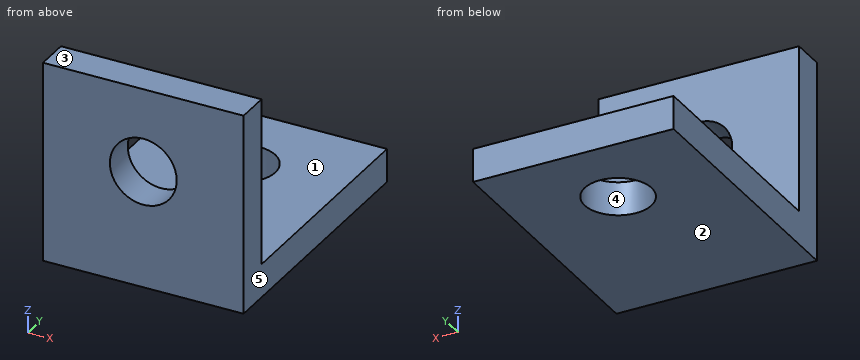
from build123d import *

# Parameters (mm, degrees)
SKETCH1_W           = 19.05
SKETCH1_H           = 19.05
BOSS_EXTRUDE1_DEPTH = 3.175
SKETCH2_W           = 19.05
SKETCH2_H           = 3.175
BOSS_EXTRUDE2_DEPTH = 22.225
CUT_EXTRUDE1_REACH  = 36.925
SKETCH3_R           = 3.175
CUT_EXTRUDE2_REACH  = 37.498
SKETCH4_R           = 3.175


with BuildPart() as part:
    # Sketch1 → Boss-Extrude1 (new body)
    with BuildSketch(Plane(origin=(0, 0, 0), x_dir=(1, 0, 0), z_dir=(0, 1, 0))):
        with Locations((9.525, -9.525)):
            Rectangle(SKETCH1_W, SKETCH1_H)
    extrude(amount=BOSS_EXTRUDE1_DEPTH)

    # Sketch2 → Boss-Extrude2 (add)
    with BuildSketch(Plane(origin=(0, 3.175, 0), x_dir=(1, 0, 0), z_dir=(0, 1, 0))):
        with Locations((9.525, -1.5875)):
            Rectangle(SKETCH2_W, SKETCH2_H)
    extrude(amount=BOSS_EXTRUDE2_DEPTH)

    # Sketch3 → Cut-Extrude1 (cut, up to next)
    with BuildSketch(Plane(origin=(0, 3.175, 0), x_dir=(1, 0, 0), z_dir=(0, 1, 0)), mode=Mode.PRIVATE) as cut_extrude1_sk1:
        with Locations(Location((9.525, -11.1125, 0), (0, 0, 270))):
            Circle(SKETCH3_R)
    cut_extrude1_tool1 = extrude(cut_extrude1_sk1.sketch, amount=-CUT_EXTRUDE1_REACH, mode=Mode.PRIVATE) & part.part
    add(cut_extrude1_tool1.solids().sort_by_distance((9.525, 3.175, 11.1125))[0], mode=Mode.SUBTRACT)

    # Sketch4 → Cut-Extrude2 (cut, up to next)
    with BuildSketch(Plane.XY.offset(3.175), mode=Mode.PRIVATE) as cut_extrude2_sk1:
        with Locations((9.525, 17.4625)):
            Circle(SKETCH4_R)
    cut_extrude2_tool1 = extrude(cut_extrude2_sk1.sketch, amount=-CUT_EXTRUDE2_REACH, mode=Mode.PRIVATE) & part.part
    add(cut_extrude2_tool1.solids().sort_by_distance((9.525, 17.4625, 3.175))[0], mode=Mode.SUBTRACT)


solid = part.part
Geometry check sheet. Reference: the model listing, model coordinates, mm. Face numbers are marked on the shaded views. A direction names the side the tool comes from. Round coordinates to 2 decimals unless told otherwise and drop trailing zeros. Write each loop counter-clockwise with the first axis right and the second up, starting at its lowest first coordinate (ties: lowest second). Pieces come first, ordered by that corner, then holes. Notation, with made-up numbers: (-1.75, 13.25) - (14.25, 13.25) arc R32 cw to (14.25, 51.25) - close; hole circle Ø6 at (80.25, -14). An arc over 180 degrees is marked (long way). One line per item, written item: value.
1. Scan lines: L1, parallel to Z at x = 13.75, y = 10.75 (3 decimals); L2, parallel to X at y = 1.25, z = 8.25. Record each from-to range of solid material in increasing order.
The answers:
L1: z = 0 to 3.175
L2: x = 0 to 8.15, 10.9 to 19.05
2. Cross-section at A-A on y = 17. Record the boundary of the cut face in (x, z) (3 decimals).
The answers:
outline: (0, 0) - (6.384, 0) - (6.384, 3.175) - (0, 3.175) - close; (12.666, 0) - (19.05, 0) - (19.05, 3.175) - (12.666, 3.175) - close
3. Depth check by flat-ended pin: pin 1 Ø8.5 at (x, y) = (9.52, 17.46) entering from +Z (3 decimals); pin 2 Ø3 at (y, z) = (6.5, 11) entering from -X; pin 3 Ø2 at (x, z) = (10, 16.5) entering from +Y (3 decimals). Enter the tip coordinate at first touch or a pass-through.
The answers:
pin 1: stops at z = 3.175
pin 2: passes through
pin 3: stops at y = 3.175
4. Cross-section at B-B on x = 7.25. Record the boundary of the cut face in (y, z) (3 decimals).
The answers:
outline: (0, 0) - (15.248, 0) - (15.248, 3.175) - (3.175, 3.175) - (3.175, 8.898) - (0, 8.898) - close; (0, 13.327) - (3.175, 13.327) - (3.175, 19.05) - (0, 19.05) - close; (19.677, 0) - (25.4, 0) - (25.4, 3.175) - (19.677, 3.175) - close
5. Set-up check for the marked faces 1 and 2: record each of +Z, -Z, +X, -X, +Y, -Y from which the full face is reachable in a straight line by a thin tool's end or side.
The answers:
face 1: +Z, +X, -X, +Y
face 2: -Z, +X, -X, +Y, -Y
6. Mould release check, pull along X, two halves, no side actions. Record for the marked faces 3, 4 and 5: released by +X, released by -X, zero draft, split by the parting line, or undercut.
The answers:
face 3: zero draft
face 4: undercut
face 5: released by +X
